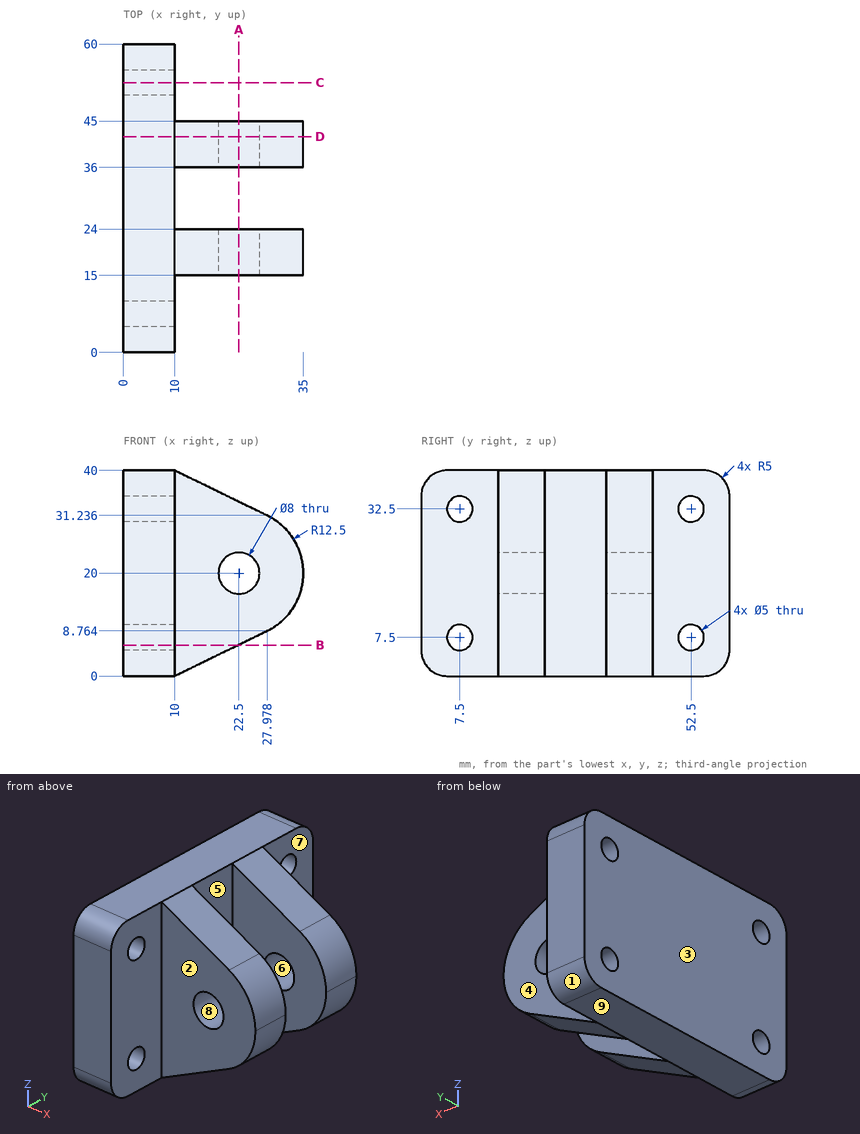
Part print with two shaded views. Sizes in mm from the minimum x, y, z corner. A direction names the side the tool comes from. Coordinates: 2 decimals unless noted, no trailing zeros. Write each loop counter-clockwise with the first axis right and the second up, starting at its lowest first coordinate (ties: lowest second). Pieces come first, ordered by that corner, then holes.
(1) Drill centre lines: line 1 (Z direction, x = 2.75, y = 52.5); line 2 (Y direction, x = 28.5, z = 17.5); line 3 (Z direction, x = 9, y = 7). Where is each one in solid material? Low to high.
(2) Cut at D-D on y = 42. List the corners of the cut face in (x, z).
(3) 3-axis set-ups, long thin cutter, end or side, ignore diameter. For the marked faces 1, 2, 3, 4 and 5: which of +Z, -Z, +X, -X, +Y, -Y reach the whole face in a straight line?
(4) Cut at C-C on y = 52.5. List the corners of the cut face in (x, z), and give its area (3 significant figures).
(5) Cut at B-B on z = 6. List the corners of the cut face in (x, y).
(6) Cut at A-A on x = 22.5. List the corners of the cut face in (y, z).
(7) Mould opens along Z. For the marked faces 6, 7, 8 and 9 say: pulls with the +Z half, pulls with the -Z half, needs draft (parallel to the pull), parting line crosses it, or undercut.
(8) Pin check, flat tips, straight feed: pin 1 Ø13 at (x, z) = (22.5, 20) entering from -Y; pin 2 Ø20 at (x, z) = (21, 10.5) entering from +Y; pin 3 Ø16.5 at (y, z) = (6, 29) entering from +X; pin 4 Ø8 at (y, z) = (39, 32.5) entering from -X. Stop position of each tip, or through.
Working result:
1. line 1: z = 0 to 5, 10 to 30, 35 to 40
1. line 2: y = 15 to 24, 36 to 45
1. line 3: z = 0 to 5.05, 9.95 to 30.05, 34.95 to 40
2. outline: (0, 0) - (10, 0) - (27.98, 8.76) arc R12.5 ccw to (35, 20) arc R12.5 ccw to (27.98, 31.24) - (10, 40) - (0, 40) - close; hole circle Ø8 at (22.5, 20)
3. face 1: -Z, +X, -X, +Y
3. face 2: +Z, -Z, +X, -Y
3. face 3: +Z, -Z, -X, +Y, -Y
3. face 4: +Z, -Z, +X, +Y
3. face 5: +Z, -Z, +X
4. outline: (0, 0) - (10, 0) - (10, 5) - (0, 5) - close; (0, 10) - (10, 10) - (10, 30) - (0, 30) - close; (0, 35) - (10, 35) - (10, 40) - (0, 40) - close
4. area: 300 mm2
5. outline: (0, 0) - (10, 0) - (10, 5.5) - (0, 5.5) - close; (0, 9.5) - (10, 9.5) - (10, 15) - (22.31, 15) - (22.31, 24) - (10, 24) - (10, 36) - (22.31, 36) - (22.31, 45) - (10, 45) - (10, 50.5) - (0, 50.5) - close; (0, 54.5) - (10, 54.5) - (10, 60) - (0, 60) - close
6. outline: (15, 6.09) - (24, 6.09) - (24, 16) - (15, 16) - close; (15, 24) - (24, 24) - (24, 33.91) - (15, 33.91) - close; (36, 6.09) - (45, 6.09) - (45, 16) - (36, 16) - close; (36, 24) - (45, 24) - (45, 33.91) - (36, 33.91) - close
7. face 6: undercut
7. face 7: needs draft
7. face 8: undercut
7. face 9: pulls with the -Z half
8. pin 1: stops at y = 15
8. pin 2: stops at y = 45
8. pin 3: stops at x = 10
8. pin 4: stops at x = 0
